Autodesk Inventor part; units mm, degrees
ref_plane "YZ Plane" through (0, 0, 0) normal (1, 0, 0) x (0, 1, 0)
ref_plane "XY Plane" through (0, 0, 0) normal (0, 0, 1) x (1, 0, 0)
sketch "BASEsc" plane through (0, 0, 0) normal (0, 1, 0) x (-1, 0, 0)
  line L0 (-29.4, -81.4) -> (29.4, -81.4)
  line L1 (37.4, -73.4) -> (37.4, 73.4)
  line L2 (29.4, 81.4) -> (-29.4, 81.4)
  line L3 (-37.4, 73.4) -> (-37.4, -73.4)
  line L4 (-37.4, -81.4) -> (37.4, 81.4) construction
  line L5 (37.4, -81.4) -> (-37.4, 81.4) construction
  arc A0 (37.4, 73.4) -> (29.4, 81.4) centre (29.4, 73.4) ccw
  arc A1 (-29.4, 81.4) -> (-37.4, 73.4) centre (-29.4, 73.4) ccw
  arc A2 (-37.4, -73.4) -> (-29.4, -81.4) centre (-29.4, -73.4) ccw
  arc A3 (29.4, -81.4) -> (37.4, -73.4) centre (29.4, -73.4) ccw
  line L6 (25.4, 74.9) -> (7.4, 74.9)
  line L7 (2.4, 69.9) -> (2.4, 43.9)
  line L8 (7.4, 38.9) -> (25.4, 38.9)
  line L9 (30.4, 43.9) -> (30.4, 69.9)
  line L10 (30.4, 74.9) -> (2.4, 38.9) construction
  line L11 (2.4, 74.9) -> (30.4, 38.9) construction
  arc A4 (30.4, 69.9) -> (25.4, 74.9) centre (25.4, 69.9) ccw
  arc A5 (7.4, 74.9) -> (2.4, 69.9) centre (7.4, 69.9) ccw
  arc A6 (25.4, 38.9) -> (30.4, 43.9) centre (25.4, 43.9) ccw
  arc A7 (2.4, 43.9) -> (7.4, 38.9) centre (7.4, 43.9) ccw
  point P0 (0, 0)
  point P1 (16.4, 56.9)
  dimension "d0" = 74.8
  dimension "d1" = 162.8
  dimension "d2" = 8
  dimension "d3" = 8
  dimension "d4" = 8
  dimension "d7" = 28
  dimension "d8" = 36
  dimension "d9" = 5
  dimension "d26" = 42.5
  dimension "d27" = 35
extrude "押し出し1" add sketch "BASEsc" along normal blind 8.3 contours A2 L3 A1 L2 A0 L1 A3 L0 | A4 L9 A6 L8 A7 L7 A5 L6
extrude "押し出し2" add sketch "BASEsc" against normal blind 1 contours A4 L9 A6 L8 A7 L7 A5 L6
sketch "スケッチ2" plane through (-37.4, 0, -73.4) normal (-1, 0, 0) x (0, 0, 1)
  line L0 (143.2215, 4.15) -> (137.7549, 4.15) construction
  line L1 (0, 8.3) -> (146.8, 8.3)
  line L2 (132.2, 3.5) -> (113.4, 3.5)
  line L3 (112.8, 4.1) -> (112.8, 4.2)
  line L4 (113.4, 4.8) -> (132.2, 4.8)
  line L5 (132.8, 4.2) -> (132.8, 4.1)
  line L6 (132.8, 3.5) -> (112.8, 4.8) construction
  line L7 (112.8, 3.5) -> (132.8, 4.8) construction
  arc A0 (132.8, 4.2) -> (132.2, 4.8) centre (132.2, 4.2) ccw
  arc A1 (132.2, 3.5) -> (132.8, 4.1) centre (132.2, 4.1) ccw
  arc A2 (112.8, 4.1) -> (113.4, 3.5) centre (113.4, 4.1) ccw
  arc A3 (113.4, 4.8) -> (112.8, 4.2) centre (113.4, 4.2) ccw
  line L8 (154.8, 0) -> (154.8, 8.3)
  line L9 (105.3, 4.6243) -> (91.8, 4.6243)
  line L10 (91.8, 4.6243) -> (91.8, 3.6757)
  line L11 (91.8, 3.6757) -> (105.3, 3.6757)
  line L12 (105.3, 3.6757) -> (105.3, 4.6243)
  line L13 (105.3, 4.6243) -> (91.8, 3.6757) construction
  line L14 (91.8, 4.6243) -> (105.3, 3.6757) construction
  point P0 (73.4, 0)
  point P1 (140.4882, 4.15)
  point P2 (122.8, 4.15)
  point P3 (112.8, 4.15)
  point P4 (98.55, 4.15)
  point P5 (105.3, 4.15)
  dimension "d12" = 4.15
  dimension "d13" = 20
  dimension "d14" = 1.3
  dimension "d15" = 0.6
  dimension "d16" = 0.6
  dimension "d17" = 42
  dimension "d18" = 7.5
  dimension "d19" = 13.5
extrude "押し出し3" add sketch "スケッチ2" along normal blind 3
sketch "スケッチ3" plane through (29.4, 0, -81.4) normal (0, 0, -1) x (-1, 0, 0)
  line L0 (-8, 0) -> (-8, 8.3)
  line L1 (66.8, 0) -> (66.8, 8.3)
  line L2 (-8, 8.3) -> (66.8, 0) construction
  line L3 (66.8, 0) -> (66.8, 8.3)
  line L4 (0, 0) -> (-8, 0)
  line L5 (66.8, 8.3) -> (-8, 0) construction
  line L6 (24.4, 6.15) -> (34.4, 6.15)
  line L7 (34.4, 6.15) -> (34.4, 2.15)
  line L8 (34.4, 2.15) -> (24.4, 2.15)
  line L9 (24.4, 2.15) -> (24.4, 6.15)
  line L10 (24.4, 6.15) -> (34.4, 2.15) construction
  line L11 (34.4, 6.15) -> (24.4, 2.15) construction
  circle A0 centre (12.4, 4.15) radius 3.5
  point P0 (29.4, 0)
  point P1 (29.4, 4.15)
  point P2 (29.4, 4.15)
  dimension "d22" = 10
  dimension "d23" = 4
  dimension "d24" = 7
  dimension "d25" = 17
extrude "押し出し4" cut sketch "スケッチ3" against normal blind 1
fillet "フィレット1" radius 1.5 8 edges at (35.0569, 8.3, -79.0569) (0, 8.3, -81.4) (-35.0569, 8.3, -79.0569) (-37.4, 8.3, 0) (-35.0569, 8.3, 79.0569) (0, 8.3, 81.4) (35.0569, 8.3, 79.0569) (37.4, 8.3, 0)
fillet "フィレット2" radius 1.5 8 edges at (-35.0569, 0, 79.0569) (0, 0, 81.4) (35.0569, 0, 79.0569) (37.4, 0, 0) (35.0569, 0, -79.0569) (0, 0, -81.4) (-35.0569, 0, -79.0569) (-37.4, 0, 0)
equation "\"BendRadius\" = Thickness"
equation "\"BendReliefWidth\" = Thickness"
equation "\"BendReliefDepth\" = 0.5 * Thickness"
equation "\"CornerReliefSize\" = 4 * Thickness"
equation "\"MinimumRemnant\" = 2 * Thickness"
equation "\"TransitionRadius\" = BendRadius"
equation "\"JacobiRadiusSize\" = BendRadius"
equation "\"GapSize\" = Thickness"
properties part number "template"
Verification items for the finished model (mm, model axes). A direction names the side the tool comes from. Round coordinates to 2 decimals unless told otherwise and drop trailing zeros. Write each loop counter-clockwise with the first axis right and the second up, starting at its lowest first coordinate (ties: lowest second). Pieces come first, ordered by that corner, then holes.
1. Section check D-D on x = -13. Enter the section's corners in (y, z), plus the area to 3 significant figures.
2. Draft check along X on faces 1 (the flat face through (0, 4, -80.4)), 2 (the cylindrical face through (-3.9, -0.49, 73.47)), 3 (the flat face through (-39, 4.8, 49)). Enter one of: +X half, -X half, draft (parallel to the pull), parting line (faces both ways), or undercut.
3. Section check B-B on x = 7.5. Enter the section's corners in (y, z).
4. Access from +Z, -Z, +X, -X, +Y, -Y to the whole of each face (thin tool, end or side, straight path). Record for faces 4 (the flat face through (-39, 3.5, 50)), 5 (the cylindrical face through (-28.97, -0.49, 73.4)), 6 (the flat face through (-39, 4.624, 25)).
5. Gauge pin test, flat ends, axial feed: P1, Ø0.8, axis at x = -19, y = -0.5, coming from the -Z side; P2, Ø0.8, axis at x = -2.5, z = -81, coming from the -Y side; P3, Ø4, axis at x = 10.5, z = 36.5, coming from the -Y side. Record the tip position at first contact, or that the pin passes through.
6. Section check C-C on z = 47.5. Enter the section's corners in (x, y).
7. Scan lines: L1, parallel to X at y = 4.15, z = -80.8; L2, parallel to X at y = 4.75, z = 29; L3, parallel to Y at x = 17, z = -80. Record each from-to range of solid material in increasing order.
8. Section check A-A on z = 24. Enter the section's corners in (x, y), plus the area to 3 significant figures.
Answer:
1. outline: (-1, 38.9) - (0, 38.9) - (0, -79.9) arc R1.5 ccw to (1.5, -81.4) - (6.8, -81.4) arc R1.5 ccw to (8.3, -79.9) - (8.3, 79.9) arc R1.5 ccw to (6.8, 81.4) - (1.5, 81.4) arc R1.5 ccw to (0, 79.9) - (0, 74.9) - (-1, 74.9) - close
1. area: 1,390 mm2
2. face 1: undercut
2. face 2: +X half
2. face 3: draft
3. outline: (0, -79.9) arc R1.5 ccw to (1.5, -81.4) - (6.8, -81.4) arc R1.5 ccw to (8.3, -79.9) - (8.3, 79.9) arc R1.5 ccw to (6.8, 81.4) - (1.5, 81.4) arc R1.5 ccw to (0, 79.9) - close
4. face 4: +Z, -Z, -X, -Y
4. face 5: +Z, -X, -Y
4. face 6: -Z, -X, +Y
5. P1: stops at z = 38.9
5. P2: stops at y = 0.17
5. P3: stops at y = 0
6. outline: (-40.4, 3.5) - (-37.4, 3.5) - (-37.4, 1.5) arc R1.5 ccw to (-35.9, 0) - (-30.4, 0) - (-30.4, -1) - (-2.4, -1) - (-2.4, 0) - (35.9, 0) arc R1.5 ccw to (37.4, 1.5) - (37.4, 6.8) arc R1.5 ccw to (35.9, 8.3) - (-35.9, 8.3) arc R1.5 ccw to (-37.4, 6.8) - (-37.4, 4.8) - (-40.4, 4.8) - close
7. L1: x = -32.44 to -5, 5 to 13.5, 20.5 to 32.44
7. L2: x = -37.4 to 37.4
7. L3: y = 0 to 8.3
8. outline: (-40.4, 3.68) - (-37.4, 3.68) - (-37.4, 1.5) arc R1.5 ccw to (-35.9, 0) - (35.9, 0) arc R1.5 ccw to (37.4, 1.5) - (37.4, 6.8) arc R1.5 ccw to (35.9, 8.3) - (-35.9, 8.3) arc R1.5 ccw to (-37.4, 6.8) - (-37.4, 4.62) - (-40.4, 4.62) - close
8. area: 622 mm2
